Geometry: final body of the model. Coordinates: model frame, mm. A direction names the side the tool comes from. Round coordinates to 2 decimals unless told otherwise and drop trailing zeros. Loops run counter-clockwise (first coordinate to the right, second up) from the corner with the lowest first, then second, coordinate; pieces in that order, holes last. Notation, with made-up numbers: (34.25, 45.5) - (83.25, 45.5) arc R29 cw to (83.25, 70.5) - close; hole circle Ø11 at (46, -14.5). An arc over 180 degrees is marked (long way). Answer as CSV lines item,"result".
Autodesk Fusion 360 part; units mm, degrees
sketch "Sketch1" plane through (0, 0, 0) normal (0, 0, 1) x (1, 0, 0)
  circle A0 centre (0, 0) radius 22.5
  circle A1 centre (0, 0) radius 20.95
  circle A2 centre (0, 0) radius 14
  dimension "d1" = 45
  dimension "d2" = 41.9
  dimension "d3" = 28
extrude "Extrude1" add sketch "Sketch1" along normal blind 8 contours A0
extrude "Extrude2" add sketch "Sketch1" along normal blind 2 contours A1
chamfer "Chamfer1" distance 1 angle 45 1 edges at (-19.5323, 7.5758, 8)
(1) Section A-A (y = 0). Output: boundary loops of the cut face in (x, z), and give its area (3 significant figures).
Findings below:
outline,"(-22.5, 0) - (-14, 0) - (-14, 2) - (-20.95, 2) - (-20.95, 7) - (-21.95, 8) - (-22.5, 8) - close; (14, 0) - (22.5, 0) - (22.5, 8) - (21.95, 8) - (20.95, 7) - (20.95, 2) - (14, 2) - close"
area,"51.6 mm2"
(2) Pin query (flat end, axial travel): P1, Ø3, axis at y = -2.5, z = 6.5, coming from the +X side; P2, Ø6, axis at x = -11.5, y = 3, coming from the +Z side; P3, Ø8, axis at x = 0.5, y = -8.5, coming from the -Z side; P4, Ø2, axis at x = 10, z = 4.5, coming from the -Y side. Return the tip coordinate at first contact, or that it passes through.
Findings below:
P1,"x = 22.48"
P2,"z = 2"
P3,"through"
P4,"y = -20.62"
(3) Material intervals for line 1 along Y through (x, z) = (0, 0.65); line 2 along Y through (x, z) = (0, 5.2); line 3 along Z through (x, y) = (8, -18), sorted ascending.
Findings below:
line 1,"-22.5 to -14, 14 to 22.5"
line 2,"-22.5 to -20.95, 20.95 to 22.5"
line 3,"0 to 2"
(4) Access query for faces 4 (the face through (4, -14, 2)), 5 (the face through (12.932, 5.362, 0.986)). Directions: +Z, -Z, +X, -X, +Y, -Y. A direction counts if a zero-diameter tool reaches every point of the face in a straight line with its end or side. Return the directions, or none.
Findings below:
face 4,"+Z"
face 5,"+Z, -Z"
(5) Draft query along X for faces 1 (the face through (-10.32, -9.69, 0)), 2 (the face through (10.382, 19.961, 3.944)), 3 (the face through (9.667, 18.586, 4.465)). Return one class per face: pulls with the +X half, pulls with the -X half, needs draft (parallel to the pull), parting line crosses it, or undercut.
Findings below:
face 1,"needs draft"
face 2,"parting line crosses it"
face 3,"undercut"
(6) Section C-C (z = 5). Output: boundary loops of the cut face in (x, y).
Findings below:
outline,"circle Ø45 at (0, 0); hole circle Ø41.9 at (0, 0)"
